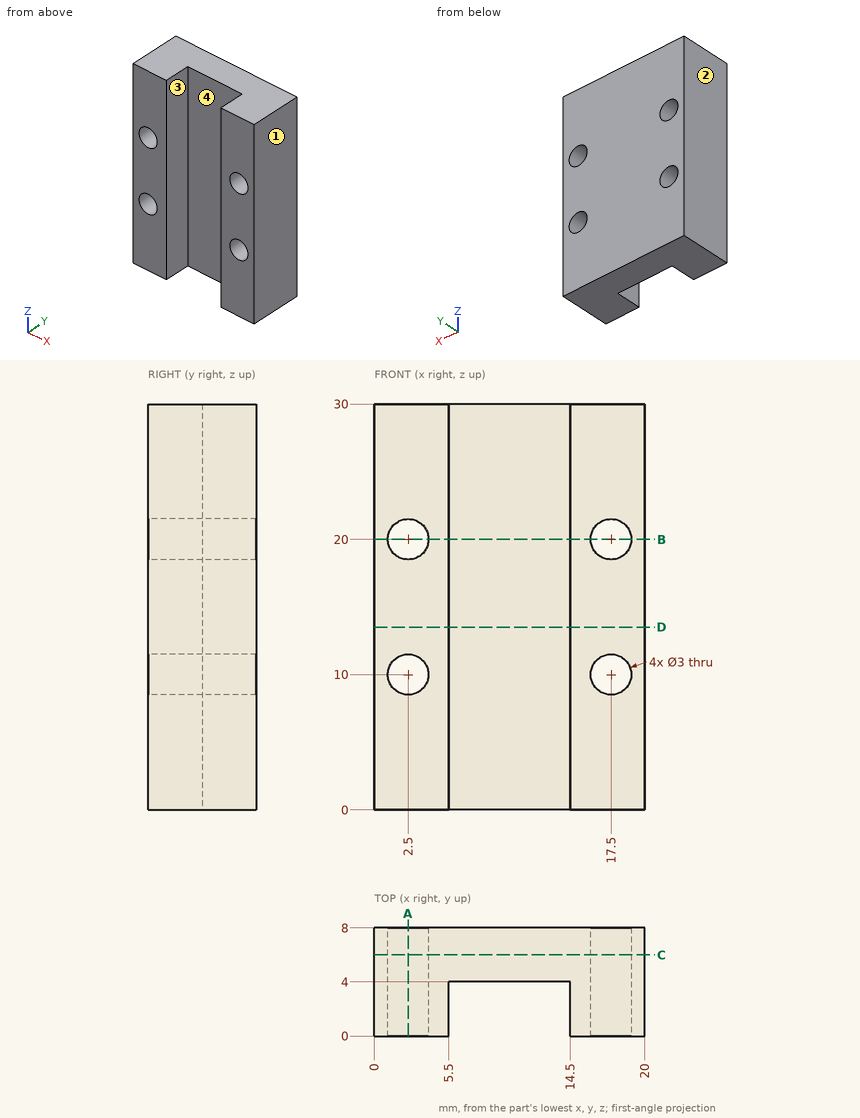
Source: three-view drawing plus pictorial views. Frame: mm from the lowest corner of the part. Coordinates: 2 decimals unless noted, no trailing zeros. Order: outer loops, then holes, each group sorted by start corner. A loop starts at its lowest first (then second) coordinate and runs counter-clockwise, first axis right, second up. Notation, with made-up numbers: M 48.5,43.25 L 68.5,43.25 A12 ccw 68.5,53.25 Z; hole C 1.5,81.5 d5. An arc over 180 degrees is marked long. Answer in a Markdown table with one row per item.
(1) Material intervals for line 1 (Z direction, x = 17.5, y = 2.5); line 2 (X direction, y = 1, z = 27.75); line 3 (X direction, y = 5.25, z = 18.75), sorted ascending. Write a range as [from, to].
Numbers:
| item | result |
|---|---|
| line 1 | z = [0, 8.5], [11.5, 18.5], [21.5, 30] |
| line 2 | x = [0, 5.5], [14.5, 20] |
| line 3 | x = [0, 1.67], [3.33, 16.67], [18.33, 20] |
(2) Section query B-B, the plane z = 20. Output: boundary loops of the cut face in (x, y).
Numbers:
| item | result |
|---|---|
| outline | M 0,0 L 1,0 L 1,8 L 0,8 Z; M 4,0 L 5.5,0 L 5.5,4 L 14.5,4 L 14.5,0 L 16,0 L 16,8 L 4,8 Z; M 19,0 L 20,0 L 20,8 L 19,8 Z |
(3) Draft query along X for the marked faces 1, 2, 3 and 4. Return one class per face: pulls with the +X half, pulls with the -X half, needs draft (parallel to the pull), parting line crosses it, or undercut.
Numbers:
| item | result |
|---|---|
| face 1 | pulls with the +X half |
| face 2 | pulls with the -X half |
| face 3 | undercut |
| face 4 | undercut |
(4) Contact query for flat-ended pins moving along their axis: pin 1 Ø4 at (x, y) = (9, 2.5) entering from -Z; pin 2 Ø6 at (x, z) = (11, 12) entering from -Y; pin 3 Ø2.5 at (x, z) = (17.5, 10) entering from -Y. Output: stop coordinate, or through.
Numbers:
| item | result |
|---|---|
| pin 1 | stops at z = 0 |
| pin 2 | stops at y = 4 |
| pin 3 | passes through |
(5) Section query A-A, the plane x = 2.5. Output: boundary loops of the cut face in (y, z), plus the area to 3 significant figures.
Numbers:
| item | result |
|---|---|
| outline | M 0,0 L 8,0 L 8,8.5 L 0,8.5 Z; M 0,11.5 L 8,11.5 L 8,18.5 L 0,18.5 Z; M 0,21.5 L 8,21.5 L 8,30 L 0,30 Z |
| area | 192 mm^2 |
(6) Section query D-D, the plane z = 13.5. Output: boundary loops of the cut face in (x, y), plus the area to 3 significant figures.
Numbers:
| item | result |
|---|---|
| outline | M 0,0 L 5.5,0 L 5.5,4 L 14.5,4 L 14.5,0 L 20,0 L 20,8 L 0,8 Z |
| area | 124 mm^2 |
(7) Section query C-C, the plane y = 6. Output: boundary loops of the cut face in (x, z), plus the area to 3 significant figures.
Numbers:
| item | result |
|---|---|
| outline | M 0,0 L 20,0 L 20,30 L 0,30 Z; hole C 2.5,10 d3; hole C 2.5,20 d3; hole C 17.5,10 d3; hole C 17.5,20 d3 |
| area | 572 mm^2 |
